from build123d import *

# Parameters (mm, degrees)
F0_W     = 35.884626
F0_H     = 49.918497
F1_DEPTH = 127
F2_R     = 16.556677


with BuildPart() as f1:
    # F0 (on Right) → F1 (new body)
    with BuildSketch(Plane.YZ):
        with Locations((112.088945, -34.705921)):
            Rectangle(F0_W, F0_H)
    extrude(amount=F1_DEPTH)

    # F2
    f2_edges = [f1.edges().sort_by_distance(p)[0] for p in [
        (63.5, 94.146632, -9.746673),
    ]]
    fillet(f2_edges, radius=F2_R)


solid = f1.part
Geometry: final body of the model. Coordinates: model frame, mm. Coordinates: 2 decimals unless noted, no trailing zeros. Order: outer loops, then holes, each group sorted by start corner. A loop starts at its lowest first (then second) coordinate and runs counter-clockwise, first axis right, second up.
1) Section C-C (z = -21.5). Return loops of the section in (x, y), then the cut area to 3 significant figures.
Result sheet:
outline: (0, 94.86) - (127, 94.86) - (127, 130.03) - (0, 130.03) - close
area: 4,470 mm2
2) Section A-A (x = 69). Return loops of the section in (y, z).
Result sheet:
outline: (94.15, -59.67) - (130.03, -59.67) - (130.03, -9.75) - (110.7, -9.75) arc R16.56 ccw to (94.15, -26.3) - close
3) Section B-B (y = 103.5). Return loops of the section in (x, z).
Result sheet:
outline: (0, -59.67) - (127, -59.67) - (127, -11.4) - (0, -11.4) - close
4) Ray query, probe 1 along Z at (x, y) = (26, 110); probe 2 along Z at (x, y) = (111, 107); probe 3 along Y at (x, z) = (86.5, -13). Return the intervals inside material, ascending.
Result sheet:
probe 1: z = -59.67 to -9.76
probe 2: z = -59.67 to -10.17
probe 3: y = 100.85 to 130.03
5) First-contact query: P1, Ø8, axis at y = 104, z = -46, coming from the -X side; P2, Ø6, axis at x = 101.5, y = 107, coming from the +Z side; P3, Ø4, axis at x = 17.5, y = 99, coming from the +Z side. Flat tips, straight axial feed; report the tip coordinate or a pass-through.
Result sheet:
P1: stops at x = 0
P2: stops at z = -9.76
P3: stops at z = -12.89
